Source: CAD feature listing. Evaluate the final solid. Frame: model axes, mm. A direction names the side the tool comes from. Give positions to 0.01 mm unless a question says otherwise; leave off trailing zeros. Order: outer loops, then holes, each group sorted by start corner. A loop starts at its lowest first (then second) coordinate and runs counter-clockwise, first axis right, second up.
1) Section B-B, the plane z = 2.1. Return loops of the section in (x, y).
2) Section A-A, the plane y = 0. Return loops of the section in (x, z), plus the area to 3 significant figures.
3) Section D-D, the plane x = 4.5. Return loops of the section in (y, z), plus the area to 3 significant figures.
4) Draft query along Y for faces 1 (the face through (3.129, -5.767, 3.246)), 2 (the face through (1.12, 1.74, 1.87)), 3 (the face through (-1.87, -0.01, 1.87)), 4 (the face through (5.5, -2.9, 0.5)). Return one class per face: released by +Y, released by -Y, zero draft, split by the parting line, or undercut.
5) Material intervals for line 1 (X direction, y = 1.5, z = 2.75); line 2 (Y direction, x = 0, z = 3.4); line 3 (Z direction, x = 2, y = -3), sorted ascending.
6) Access query for faces 5 (the face through (-3, 0, 3.5)), 6 (the face through (1, 2, 0)), 7 (the face through (-2.03, 1.24, 1.87)). Directions: +Z, -Z, +X, -X, +Y, -Y. A direction counts if a zero-diameter tool reaches every point of the face in a straight line with its end or side. Return the directions, or none.
7) Section C-C, the plane x = 0. Return loops of the section in (y, z), plus the area to 3 significant figures.
8) First-contact query: P1, Ø1.5, axis at y = 0.5, z = 2, coming from the +X side; P2, Ø0.6, axis at y = -2, z = 1, coming from the -X side; P3, Ø2, axis at x = -4, y = 5, coming from the +Z side. Flat tips, straight axial feed; report the tip coordinate or a pass-through.
```python
from build123d import *

# Parameters (mm, degrees)
SKETCH1_R           = 6.5
BOSS_EXTRUDE1_DEPTH = 3.5
SKETCH3_R           = 3
BOSS_EXTRUDE2_DEPTH = 0.3
SKETCH4_R           = 6.5
SKETCH4_R_2         = 6
CUT_EXTRUDE1_DEPTH  = 2.5


with BuildPart() as part:
    # Sketch1 → Boss-Extrude1 (new body)
    with BuildSketch(Plane.XY):
        with Locations((0.129947127, 0)):
            Circle(SKETCH1_R)
        with BuildLine():
            Line((-0.370052873, 1.936491673), (-0.370052873, 2.439282681))
            ThreePointArc((-0.370052873, 2.439282681), (0.129947127, 2.49), (0.629947127, 2.439282681))
            Line((0.629947127, 2.439282681), (0.629947127, 1.936491673))
            ThreePointArc((0.629947127, 1.936491673), (1.129947127, 1.732050808), (1.55699811, 1.401258538))
            Line((1.55699811, 1.401258538), (1.992427896, 1.652654043))
            ThreePointArc((1.992427896, 1.652654043), (2.286350382, 1.245), (2.492427896, 0.786628639))
            Line((2.492427896, 0.786628639), (2.05699811, 0.535233135))
            ThreePointArc((2.05699811, 0.535233135), (2.129947127, 0), (2.05699811, -0.535233135))
            Line((2.05699811, -0.535233135), (2.492427896, -0.786628639))
            ThreePointArc((2.492427896, -0.786628639), (2.286350382, -1.245), (1.992427896, -1.652654043))
            Line((1.992427896, -1.652654043), (1.55699811, -1.401258538))
            ThreePointArc((1.55699811, -1.401258538), (1.129947127, -1.732050808), (0.629947127, -1.936491673))
            Line((0.629947127, -1.936491673), (0.629947127, -2.439282681))
            ThreePointArc((0.629947127, -2.439282681), (0.129947127, -2.49), (-0.370052873, -2.439282681))
            Line((-0.370052873, -2.439282681), (-0.370052873, -1.936491673))
            ThreePointArc((-0.370052873, -1.936491673), (-0.870052873, -1.732050808), (-1.297103856, -1.401258538))
            Line((-1.297103856, -1.401258538), (-1.732533642, -1.652654043))
            ThreePointArc((-1.732533642, -1.652654043), (-2.026456129, -1.245), (-2.232533642, -0.786628639))
            Line((-2.232533642, -0.786628639), (-1.797103856, -0.535233135))
            ThreePointArc((-1.797103856, -0.535233135), (-1.870052873, 0), (-1.797103856, 0.535233135))
            Line((-1.797103856, 0.535233135), (-2.232533642, 0.786628639))
            ThreePointArc((-2.232533642, 0.786628639), (-2.026456129, 1.245), (-1.732533642, 1.652654043))
            Line((-1.732533642, 1.652654043), (-1.297103856, 1.401258538))
            ThreePointArc((-1.297103856, 1.401258538), (-0.870052873, 1.732050808), (-0.370052873, 1.936491673))
        make_face(mode=Mode.SUBTRACT)
    extrude(amount=BOSS_EXTRUDE1_DEPTH)

    # Sketch3 → Boss-Extrude2 (add)
    with BuildSketch(Plane.XY.offset(3.5)):
        with Locations((0.314947127, 0)):
            Circle(SKETCH3_R)
        with BuildLine():
            Line((0.629947127, 2.439282681), (0.629947127, 1.936491673))
            ThreePointArc((0.629947127, 1.936491673), (1.129947127, 1.732050808), (1.55699811, 1.401258538))
            Line((1.55699811, 1.401258538), (1.992427896, 1.652654043))
            ThreePointArc((1.992427896, 1.652654043), (2.286350382, 1.245), (2.492427896, 0.786628639))
            Line((2.492427896, 0.786628639), (2.05699811, 0.535233135))
            ThreePointArc((2.05699811, 0.535233135), (2.129947127, 0), (2.05699811, -0.535233135))
            Line((2.05699811, -0.535233135), (2.492427896, -0.786628639))
            ThreePointArc((2.492427896, -0.786628639), (2.286350382, -1.245), (1.992427896, -1.652654043))
            Line((1.992427896, -1.652654043), (1.55699811, -1.401258538))
            ThreePointArc((1.55699811, -1.401258538), (1.129947127, -1.732050808), (0.629947127, -1.936491673))
            Line((0.629947127, -1.936491673), (0.629947127, -2.439282681))
            ThreePointArc((0.629947127, -2.439282681), (0.129947127, -2.49), (-0.370052873, -2.439282681))
            Line((-0.370052873, -2.439282681), (-0.370052873, -1.936491673))
            ThreePointArc((-0.370052873, -1.936491673), (-0.870052873, -1.732050808), (-1.297103856, -1.401258538))
            Line((-1.297103856, -1.401258538), (-1.732533642, -1.652654043))
            ThreePointArc((-1.732533642, -1.652654043), (-2.026456129, -1.245), (-2.232533642, -0.786628639))
            Line((-2.232533642, -0.786628639), (-1.797103856, -0.535233135))
            ThreePointArc((-1.797103856, -0.535233135), (-1.870052873, 0), (-1.797103856, 0.535233135))
            Line((-1.797103856, 0.535233135), (-2.232533642, 0.786628639))
            ThreePointArc((-2.232533642, 0.786628639), (-2.026456129, 1.245), (-1.732533642, 1.652654043))
            Line((-1.732533642, 1.652654043), (-1.297103856, 1.401258538))
            ThreePointArc((-1.297103856, 1.401258538), (-0.870052873, 1.732050808), (-0.370052873, 1.936491673))
            Line((-0.370052873, 1.936491673), (-0.370052873, 2.439282681))
            ThreePointArc((-0.370052873, 2.439282681), (0.129947127, 2.49), (0.629947127, 2.439282681))
        make_face(mode=Mode.SUBTRACT)
    extrude(amount=BOSS_EXTRUDE2_DEPTH)

    # Sketch4 → Cut-Extrude1 (cut)
    with BuildSketch(Plane(origin=(0, 0, 0.5), x_dir=(-1, 0, 0), z_dir=(0, 0, -1))):
        with Locations((-0.129947127, 0)):
            Circle(SKETCH4_R)
        Circle(SKETCH4_R_2, mode=Mode.SUBTRACT)
    extrude(amount=-CUT_EXTRUDE1_DEPTH, mode=Mode.SUBTRACT)


solid = part.part
```
From the geometry:
1. outline: circle Ø12 at (0, 0); hole (-2.23, -0.79) arc R2.49 ccw to (-1.73, -1.65) - (-1.3, -1.4) arc R2 ccw to (-0.37, -1.94) - (-0.37, -2.44) arc R2.49 ccw to (0.63, -2.44) - (0.63, -1.94) arc R2 ccw to (1.56, -1.4) - (1.99, -1.65) arc R2.49 ccw to (2.49, -0.79) - (2.06, -0.54) arc R2 ccw to (2.06, 0.54) - (2.49, 0.79) arc R2.49 ccw to (1.99, 1.65) - (1.56, 1.4) arc R2 ccw to (0.63, 1.94) - (0.63, 2.44) arc R2.49 ccw to (-0.37, 2.44) - (-0.37, 1.94) arc R2 ccw to (-1.3, 1.4) - (-1.73, 1.65) arc R2.49 ccw to (-2.23, 0.79) - (-1.8, 0.54) arc R2 ccw to (-1.8, -0.54) - close
2. outline: (-6.37, 0) - (-1.87, 0) - (-1.87, 3.8) - (-2.69, 3.8) - (-2.69, 3.5) - (-6.37, 3.5) - (-6.37, 3) - (-6, 3) - (-6, 0.5) - (-6.37, 0.5) - close; (2.13, 0) - (6.63, 0) - (6.63, 0.5) - (6, 0.5) - (6, 3) - (6.63, 3) - (6.63, 3.5) - (3.31, 3.5) - (3.31, 3.8) - (2.13, 3.8) - close
2. area: 29.6 mm2
3. outline: (-4.81, 0) - (4.81, 0) - (4.81, 0.5) - (3.97, 0.5) - (3.97, 3) - (4.81, 3) - (4.81, 3.5) - (-4.81, 3.5) - (-4.81, 3) - (-3.97, 3) - (-3.97, 0.5) - (-4.81, 0.5) - close
3. area: 29.5 mm2
4. face 1: split by the parting line
4. face 2: undercut
4. face 3: undercut
4. face 4: zero draft
5. line 1: x = -5.81 to -1.86, -1.47 to -1.19, 1.45 to 1.73, 2.12 to 5.81
5. line 2: y = -6.5 to -2.49, 2.49 to 6.5
5. line 3: z = 0 to 3.5
6. face 5: +Z
6. face 6: -Z, +X, -X, +Y, -Y
6. face 7: +Z, -Z
7. outline: (-6.5, 0) - (-2.49, 0) - (-2.49, 3.8) - (-2.98, 3.8) - (-2.98, 3.5) - (-6.5, 3.5) - (-6.5, 3) - (-6, 3) - (-6, 0.5) - (-6.5, 0.5) - close; (2.49, 0) - (6.5, 0) - (6.5, 0.5) - (6, 0.5) - (6, 3) - (6.5, 3) - (6.5, 3.5) - (2.98, 3.5) - (2.98, 3.8) - (2.49, 3.8) - close
7. area: 25.9 mm2
8. P1: stops at x = 6
8. P2: stops at x = -5.75
8. P3: stops at z = 3.5
